from build123d import *

# Parameters (mm, degrees)
F0_R     = 1.8288
F0_R_2   = 3.175
F1_DEPTH = 5.588
F2_R     = 2


# Not quite as in the source:
# - a feature names something its author has since deleted; it is built from what else it names


with BuildPart() as f1:
    # F0 (on Right) → F1 (new body)
    with BuildSketch(Plane.YZ):
        with BuildLine():
            ThreePointArc((59, -22), (69.6794919243, 0), (59, 22))
            Line((59, 22), (-59, 22))
            ThreePointArc((-59, 22), (-69.6794919243, 0), (-59, -22))
            Line((-59, -22), (59, -22))
        make_face()
        with Locations((-65, -6.35)):
            Circle(F0_R, mode=Mode.SUBTRACT)
        with Locations((0, -6.35)):
            Circle(F0_R_2, mode=Mode.SUBTRACT)
        with Locations((65, -6.35)):
            Circle(F0_R, mode=Mode.SUBTRACT)
        with BuildLine():
            ThreePointArc((-30.91, -11.6189500386), (-41.91, -16), (-52.91, -11.6189500386))
            Line((-52.91, -11.6189500386), (-52.91, 11.6189500386))
            ThreePointArc((-52.91, 11.6189500386), (-41.91, 16), (-30.91, 11.6189500386))
            Line((-30.91, 11.6189500386), (-30.91, -11.6189500386))
        make_face(mode=Mode.SUBTRACT)
        with Locations((-65, 6.35)):
            Circle(F0_R, mode=Mode.SUBTRACT)
        with BuildLine():
            ThreePointArc((-27.51, 11.6189500386), (-16.51, 16), (-5.51, 11.6189500386))
            Line((-5.51, 11.6189500386), (-5.51, -11.6189500386))
            ThreePointArc((-5.51, -11.6189500386), (-16.51, -16), (-27.51, -11.6189500386))
            Line((-27.51, -11.6189500386), (-27.51, 11.6189500386))
        make_face(mode=Mode.SUBTRACT)
        with BuildLine():
            ThreePointArc((27.51, -11.6189500386), (16.51, -16), (5.51, -11.6189500386))
            Line((5.51, -11.6189500386), (5.51, 11.6189500386))
            ThreePointArc((5.51, 11.6189500386), (16.51, 16), (27.51, 11.6189500386))
            Line((27.51, 11.6189500386), (27.51, -11.6189500386))
        make_face(mode=Mode.SUBTRACT)
        with Locations((0, 6.35)):
            Circle(F0_R_2, mode=Mode.SUBTRACT)
        with BuildLine():
            ThreePointArc((52.91, -11.6189500386), (41.91, -16), (30.91, -11.6189500386))
            Line((30.91, -11.6189500386), (30.91, 11.6189500386))
            ThreePointArc((30.91, 11.6189500386), (41.91, 16), (52.91, 11.6189500386))
            Line((52.91, 11.6189500386), (52.91, -11.6189500386))
        make_face(mode=Mode.SUBTRACT)
        with Locations((65, 6.35)):
            Circle(F0_R, mode=Mode.SUBTRACT)
    extrude(amount=F1_DEPTH)

    # F2
    f2_edges = [f1.edges().sort_by_distance(p)[0] for p in [
        (2.794, -5.51, 11.61895),
        (2.794, 52.91, 11.61895),
        (2.794, 5.51, -11.61895),
        (2.794, 5.51, 11.61895),
        (2.794, -52.91, -11.61895),
        (2.794, -52.91, 11.61895),
        (2.794, -5.51, -11.61895),
        (2.794, 52.91, -11.61895),
        (2.794, -30.91, -11.61895),
        (2.794, -30.91, 11.61895),
        (2.794, -27.51, -11.61895),
        (2.794, -27.51, 11.61895),
        (2.794, 27.51, 11.61895),
        (2.794, 27.51, -11.61895),
        (2.794, 30.91, 11.61895),
        (2.794, 30.91, -11.61895),
    ]]
    fillet(f2_edges, radius=F2_R)


solid = f1.part
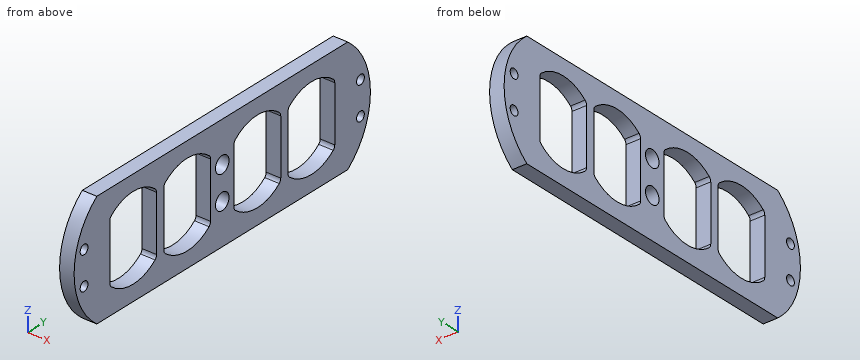
Geometry check sheet. Reference: the model listing, model coordinates, mm. Give positions to 0.01 mm unless a question says otherwise; leave off trailing zeros. Loops run counter-clockwise (first coordinate to the right, second up) from the corner with the lowest first, then second, coordinate; pieces in that order, holes last. Notation, with made-up numbers: M -26,87.25 L 32,87.25 A16 cw 32,113.25 Z; hole C 37,-16.75 d1. An arc over 180 degrees is marked long. Answer as a JSON object with one key per item and string values. Group by question number.
Item 1: Sectioned sample at A-A on y = -65. Record the boundary of the cut face in (x, z), plus the area to 3 significant figures.
Item 2: Gauge pin test, flat ends, axial feed: pin 1 (3.5 mm diameter, centred on y = 65, z = -6.35, fed in from +X); pin 2 (3 mm diameter, centred on x = 1.5, z = 1, fed in from -Y). Record the tip position at first contact, or that the pin passes through.
Item 3: Material ranges on L1, parallel to Z at x = 4.15, y = 0 (3 decimals); L2, parallel to Y at x = 4.45, z = 0.5; L3, parallel to Z at x = 0.9, y = 1, recorded low to high.
Item 4: Sectioned sample at C-C on y = 49. Record the boundary of the cut face in (x, z), plus the area to 3 significant figures.
Item 5: Sectioned sample at B-B on z = 6.35. Give the number of separate pieces and of enclosed holes in the cut face, plus the area to 3 significant figures.
Findings below:
{
 "1": {"outline": "M 0,-15.5 L 5.59,-15.5 L 5.59,-8.18 L 0,-8.18 Z; M 0,-4.52 L 5.59,-4.52 L 5.59,4.52 L 0,4.52 Z; M 0,8.18 L 5.59,8.18 L 5.59,15.5 L 0,15.5 Z", "area": "132 mm2"},
 "2": {"pin 1": "through", "pin 2": "y = -69.68"},
 "3": {"L1": "-22 to -9.525, -3.175 to 3.175, 9.525 to 22", "L2": "-69.68 to -52.91, -30.91 to -27.51, -5.51 to 5.51, 27.51 to 30.91, 52.91 to 69.68", "L3": "-22 to -9.36, -3.34 to 3.34, 9.36 to 22"},
 "4": {"outline": "M 0,-22 L 5.59,-22 L 5.59,-14.34 L 0,-14.34 Z; M 0,14.34 L 5.59,14.34 L 5.59,22 L 0,22 Z", "area": "85.6 mm2"},
 "5": {"separate pieces": "8", "enclosed holes": "0", "area": "202 mm2"}
}
